```python
from build123d import *

# Parameters (mm, degrees)
F0_R      = 1.25
F0_R_2    = 12
F1_DEPTH  = 2.3
F2_DEPTH  = 5.1
F3_W      = 14.9775519967
F3_H      = 15.6408976763
F3_W_2    = 4.8427809961
F3_H_2    = 1.104
F4_DEPTH  = 1
F5_DEPTH  = 3
F6_W      = 14.5
F6_H      = 16
F7_DEPTH  = 28
F8_W      = 4.4338763691
F8_H      = 4.8907462656
F9_DEPTH  = 8
F10_DEPTH = 30.1


with BuildPart() as f1:
    # F0 (on Front) → F1 (new body)
    with BuildSketch(Plane.XZ):
        with BuildLine():
            ThreePointArc((13, 12), (11.9748737342, 14.4748737342), (9.5, 15.5))
            Line((9.5, 15.5), (-9.5, 15.5))
            ThreePointArc((-9.5, 15.5), (-11.9748737342, 14.4748737342), (-13, 12))
            Line((-13, 12), (-13, -12))
            ThreePointArc((-13, -12), (-11.9748737342, -14.4748737342), (-9.5, -15.5))
            Line((-9.5, -15.5), (9.5, -15.5))
            ThreePointArc((9.5, -15.5), (11.9748737342, -14.4748737342), (13, -12))
            Line((13, -12), (13, 12))
        make_face()
        with Locations((9.5, -12)):
            Circle(F0_R, mode=Mode.SUBTRACT)
        with Locations((-9.5, 12)):
            Circle(F0_R, mode=Mode.SUBTRACT)
        Circle(F0_R_2, mode=Mode.SUBTRACT)
        Circle(F0_R_2)
    extrude(amount=F1_DEPTH)

    # F0 (on Front) → F2 (join)
    with BuildSketch(Plane.XZ):
        Circle(F0_R_2)
    extrude(amount=F2_DEPTH)

    # F3 (on face) → F4 (cut)
    with BuildSketch(Plane.XZ.offset(5.1)):
        Rectangle(F3_W, F3_H)
        Polygon((-4.5, 3.2868520357), (4.5, 3.2868520357), (4.5, -3.2868520357), (2.4213904981, -3.2868520357), (2.4213904981, -4.3908520357), (-2.4213904981, -4.3908520357), (-2.4213904981, -3.2868520357), (-4.5, -3.2868520357), align=None, mode=Mode.SUBTRACT)
        Polygon((4.5, -3.2868520357), (4.5, 3.2868520357), (-4.5, 3.2868520357), (-4.5, -3.2868520357), (-2.4213904981, -3.2868520357), (-2.4213904981, -2.1828520357), (2.4213904981, -2.1828520357), (2.4213904981, -3.2868520357), align=None)
        with Locations((0, -2.7348520357)):
            Rectangle(F3_W_2, F3_H_2)
        with Locations((0, -3.8388520357)):
            Rectangle(F3_W_2, F3_H_2)
    extrude(amount=-F4_DEPTH, mode=Mode.SUBTRACT)

    # F3 (on face) → F5 (cut)
    with BuildSketch(Plane.XZ.offset(5.1)):
        Polygon((4.5, -3.2868520357), (4.5, 3.2868520357), (-4.5, 3.2868520357), (-4.5, -3.2868520357), (-2.4213904981, -3.2868520357), (-2.4213904981, -2.1828520357), (2.4213904981, -2.1828520357), (2.4213904981, -3.2868520357), align=None)
        with Locations((0, -2.7348520357)):
            Rectangle(F3_W_2, F3_H_2)
        with Locations((0, -3.8388520357)):
            Rectangle(F3_W_2, F3_H_2)
    extrude(amount=-F5_DEPTH, mode=Mode.SUBTRACT)

    # F6 (on face) → F7 (join)
    with BuildSketch(Plane(origin=(0, 0, 0), x_dir=(-1, 0, 0), z_dir=(0, 1, 0))):
        Rectangle(F6_W, F6_H)
    extrude(amount=F7_DEPTH)

    # F8 (on face) → F9 (join)
    with BuildSketch(Plane(origin=(0, 0, 0), x_dir=(-1, 0, 0), z_dir=(0, 1, 0))):
        with Locations((0, 8)):
            Rectangle(F8_W, F8_H)
    extrude(amount=F9_DEPTH)

    # F10 (cut, through all): a face of the model
    f10_faces = [f1.faces().sort_by_distance(p)[0] for p in [
        (0, -2.1, -0.3181557698),
    ]]
    extrude(f10_faces, amount=-F10_DEPTH, mode=Mode.SUBTRACT)


solid = f1.part
```
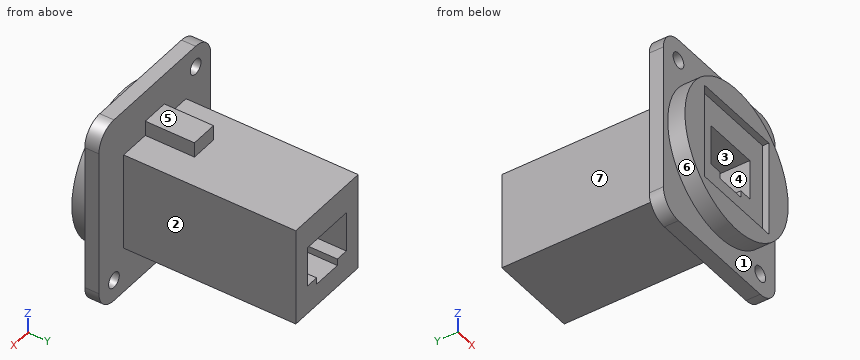
Part model, mm, in its own coordinate system. Face numbers are marked on the shaded views. A direction names the side the tool comes from. Give positions to 0.01 mm unless a question says otherwise; leave off trailing zeros. Write each loop counter-clockwise with the first axis right and the second up, starting at its lowest first coordinate (ties: lowest second). Pieces come first, ordered by that corner, then holes. Notation, with made-up numbers: (-1, -20.75) -> (10, -20.75) arc R13 ccw to (10, -13.75) -> close; hole circle Ø8 at (68.5, -13). An arc over 180 degrees is marked (long way). Put each result on its own line as item: value. Start each with the question number.
Item 1: Cut at C-C (y = 6.5). List the corners of the cut face in (x, z), then the cut area to 3 significant figures.
Item 2: Cut at D-D (x = -5.25). List the corners of the cut face in (y, z), then the cut area to 3 significant figures.
Item 3: Wall check: L1, parallel to Z at x = -9.5, y = -1; L2, parallel to Z at x = 9.5, y = -0.8; L3, parallel to Y at x = 11.5, z = 11. Give the ranges that are in metal, low to high. Write a range as [from, to].
Item 4: Which spindle directions (+Z, -Z, +X, -X, +Y, -Y) get a long thin tool onto all of the face, cutting with end or side? Do the marked faces 1, 2 and 3. Say none if no direction does.
Item 5: Cut at A-A (x = 0). List the corners of the cut face in (y, z), then the cut area to 3 significant figures.
Item 6: Pull direction Z, two halves, no side cores. Call the marked faces 4, 5, 6 and 7: pulls with the +Z half, pulls with the -Z half, needs draft (parallel to the pull), parting line crosses it, or undercut.
Item 7: Pin check, flat tips, straight feed: pin 1 Ø13 at (x, z) = (3, 0.5) entering from -Y; pin 2 Ø5 at (y, z) = (16.5, -9) entering from +X; pin 3 Ø4 at (x, y) = (-4.5, 8) entering from -Z; pin 4 Ø1 at (x, y) = (3, 2) entering from +Z. Stop position of each tip, or through.
Item 8: Cut at B-B (z = 0). List the corners of the cut face in (x, y), then the cut area to 3 significant figures.
Answer list:
1. outline: (-7.25, -8) -> (7.25, -8) -> (7.25, 8) -> (2.22, 8) -> (2.22, 10.45) -> (-2.22, 10.45) -> (-2.22, 8) -> (-7.25, 8) -> close; hole (-4.5, -3.29) -> (-2.42, -3.29) -> (-2.42, -4.39) -> (2.42, -4.39) -> (2.42, -3.29) -> (4.5, -3.29) -> (4.5, 3.29) -> (-4.5, 3.29) -> close
1. area: 178 mm2
2. outline: (-5.1, -10.79) -> (-2.3, -10.79) -> (-2.3, -15.5) -> (0, -15.5) -> (0, -8) -> (28, -8) -> (28, 8) -> (0, 8) -> (0, 15.5) -> (-2.3, 15.5) -> (-2.3, 10.79) -> (-5.1, 10.79) -> (-5.1, 7.82) -> (-4.1, 7.82) -> (-4.1, -7.82) -> (-5.1, -7.82) -> close
2. area: 564 mm2
3. L1: z = [-15.5, 10.75], [13.25, 15.5]
3. L2: z = [-15.5, -13.25], [-10.75, 15.5]
3. L3: y = [-2.3, 0]
4. face 1: -Y
4. face 2: +Z, -Z, +X, +Y
4. face 3: +Y, -Y
5. outline: (-5.1, -12) -> (-2.3, -12) -> (-2.3, -15.5) -> (0, -15.5) -> (0, -8) -> (28, -8) -> (28, -4.39) -> (-4.1, -4.39) -> (-4.1, -7.82) -> (-5.1, -7.82) -> close; (-5.1, 7.82) -> (-4.1, 7.82) -> (-4.1, 3.29) -> (28, 3.29) -> (28, 8) -> (8, 8) -> (8, 10.45) -> (0, 10.45) -> (0, 15.5) -> (-2.3, 15.5) -> (-2.3, 12) -> (-5.1, 12) -> close
5. area: 344 mm2
6. face 4: undercut
6. face 5: pulls with the +Z half
6. face 6: parting line crosses it
6. face 7: needs draft
7. pin 1: stops at y = -5.1
7. pin 2: stops at x = 7.25
7. pin 3: stops at z = -8
7. pin 4: stops at z = 8
8. outline: (-13, -2.3) -> (-12, -2.3) -> (-12, -5.1) -> (-7.49, -5.1) -> (-7.49, -4.1) -> (-4.5, -4.1) -> (-4.5, 28) -> (-7.25, 28) -> (-7.25, 0) -> (-13, 0) -> close; (4.5, -4.1) -> (7.49, -4.1) -> (7.49, -5.1) -> (12, -5.1) -> (12, -2.3) -> (13, -2.3) -> (13, 0) -> (7.25, 0) -> (7.25, 28) -> (4.5, 28) -> close
8. area: 229 mm2
